from build123d import *

# Parameters (mm, degrees)
F1_DEPTH = 63.5
F2_DEPTH = 25.4
F3_DEPTH = 12.7
F5_R     = 5.08


with BuildPart() as f1:
    # F0 (on Front) → F1 (new body, symmetric)
    with BuildSketch(Plane.XZ):
        Polygon((-41.275, 9.525), (-41.275, -9.525), (41.275, -9.525), (41.275, 9.525), (22.225, 9.525), align=None)
    extrude(amount=F1_DEPTH, both=True)

    # F0 (on Front) → F2 (join, symmetric)
    with BuildSketch(Plane.XZ):
        with BuildLine():
            Line((22.225, 9.525), (41.275, 9.525))
            Line((41.275, 9.525), (41.275, 27.0002))
            ThreePointArc((41.275, 27.0002), (45.92468, 38.22552), (57.15, 42.8752))
            Line((57.15, 42.8752), (60.325, 42.8752))
            Line((60.325, 42.8752), (60.325, 61.9252))
            Line((60.325, 61.9252), (57.15, 61.9252))
            ThreePointArc((57.15, 61.9252), (32.454296, 51.695904), (22.225, 27.0002))
            Line((22.225, 27.0002), (22.225, 9.525))
        make_face()
        Polygon((77.207536, 61.9252), (60.325, 61.9252), (60.325, 42.8752), (77.207536, 42.8752), (85.725, 42.8752), (85.725, 61.9252), align=None)
    extrude(amount=F2_DEPTH, both=True)

    # F0 (on Front) → F3 (join, symmetric)
    with BuildSketch(Plane.XZ):
        with BuildLine():
            add(Edge.make_bspline(
                [(-41.275, 9.525), (-40.73476, 34.741372), (14.03527, 61.9252), (57.15, 61.9252)],
                knots=[0, 0, 0, 0, 111.504536, 111.504536, 111.504536, 111.504536], degree=3))
            Line((-41.275, 9.525), (22.225, 9.525))
            Line((22.225, 9.525), (22.225, 27.0002))
            ThreePointArc((22.225, 27.0002), (32.454296, 51.695904), (57.15, 61.9252))
        make_face()
    extrude(amount=F3_DEPTH, both=True)

    # F0 (on Front) → F4 (revolve)
    with BuildSketch(Plane.XZ):
        Polygon((111.125, 66.675), (85.725, 66.675), (85.725, 61.9252), (85.725, 42.8752), (85.725, 38.1), (111.125, 38.1), align=None)
    revolve(axis=Axis((85.725, 0, 52.3875), (0, 0, -1)))

    # F5
    f5_edges = [f1.edges().sort_by_distance(p)[0] for p in [
        (41.275, -63.5, 0),
        (-41.275, -63.5, 0),
        (41.275, 63.5, 0),
        (-41.275, 63.5, 0),
    ]]
    fillet(f5_edges, radius=F5_R)


solid = f1.part
For this review, take the finished solid that the model builds, in its own axes (mm). A direction names the side the tool comes from. Coordinates: 2 decimals unless noted, no trailing zeros. Loops run counter-clockwise (first coordinate to the right, second up) from the corner with the lowest first, then second, coordinate; pieces in that order, holes last. Notation, with made-up numbers: (-18.5, 49.5) - (24.5, 49.5) arc R9 ccw to (24.5, 61.5) - close; hole circle Ø10 at (-20, 58). An arc over 180 degrees is marked (long way). Return JSON: item names as keys, results as strings.
Item 1: For line 1 (Y direction, x = 53, z = 58); line 2 (Z direction, x = 19.5, y = -23) (3 decimals); line 3 (X direction, y = 15.5, z = 41.5), list the stretches that pass through material, from the lowest coordinate up.
Determined:
{"line 1": "y = -25.4 to 25.4", "line 2": "z = -9.525 to 9.525", "line 3": "x = 25.38 to 50.69, 65.6 to 105.85"}
Item 2: For faces 1 (the flat face through (60, -2, 61.925)), 2 (the flat face through (22.225, 19, 18)), 3 (the flat face through (-2, -12.7, 30)), 4 (the flat face through (41.275, -1, 4)), list the 3-axis set-ups (+Z, -Z, +X, -X, +Y, -Y) from which the entire face can be reached by the end or side of a thin tool; tool diameter is ignored.
Determined:
{"face 1": "+Z, -X", "face 2": "+Z, -X, +Y", "face 3": "+Z, -X, -Y", "face 4": "-Z, +X, +Y, -Y"}
Item 3: Take a section at C-C (y = 52). Give the boundary of the cut face in (x, z) (3 decimals).
Determined:
{"outline": "(-41.275, -9.525) - (41.275, -9.525) - (41.275, 9.525) - (-41.275, 9.525) - close"}
Item 4: Take a section at A-A (x = 70). Give the boundary of the cut face in (y, z) (3 decimals), then the cut area to 3 significant figures.
Determined:
{"outline": "(-25.4, 42.875) - (-19.947, 42.875) - (-19.947, 38.1) - (19.947, 38.1) - (19.947, 42.875) - (25.4, 42.875) - (25.4, 61.925) - (19.947, 61.925) - (19.947, 66.675) - (-19.947, 66.675) - (-19.947, 61.925) - (-25.4, 61.925) - close", "area": "1,350 mm2"}
Item 5: Take a section at B-B (z = -4). Give the boundary of the cut face in (x, y) (3 decimals).
Determined:
{"outline": "(-41.275, -58.42) arc R5.08 ccw to (-36.195, -63.5) - (36.195, -63.5) arc R5.08 ccw to (41.275, -58.42) - (41.275, 58.42) arc R5.08 ccw to (36.195, 63.5) - (-36.195, 63.5) arc R5.08 ccw to (-41.275, 58.42) - close"}
Item 6: Mouldability with a two-part tool opening along X and no side actions: class faces 5 (the flat face through (60, 2, 42.875)), 6 (the cylindrical face through (39.8, -62, 0.1)), 7 (the flat face through (-1, -1, -9.525)), 8 (the cylindrical face through (-39.8, 62, -0.1)) as pulls with the +X half, pulls with the -X half, needs draft (parallel to the pull), parting line crosses it, or undercut.
Determined:
{"face 5": "undercut", "face 6": "pulls with the +X half", "face 7": "needs draft", "face 8": "pulls with the -X half"}
Item 7: Insertion check: pin 1 (3 mm diameter, centred on x = 36.5, y = -48.5, fed in from +Z) (3 decimals); pin 2 (1.5 mm diameter, centred on x = 58.5, y = -3, fed in from -Z); pin 3 (15 mm diameter, centred on x = 88.5, y = 3.5, fed in from -Z). Each pin has a flat end and moves straight along its axis. Give the tip position at first contact, or say it passes through.
Determined:
{"pin 1": "stops at z = 9.525", "pin 2": "stops at z = 42.88", "pin 3": "stops at z = 38.1"}
